Design review of the part built by this model. Coordinates are the model's own, in mm. Coordinates: 2 decimals unless noted, no trailing zeros. Write each loop counter-clockwise with the first axis right and the second up, starting at its lowest first coordinate (ties: lowest second). Pieces come first, ordered by that corner, then holes.
Q1. Add section B-B, the plane x = -28. Give the boundary of the cut face in (y, z), plus the area to 3 significant figures.
Q2. Clearance check with flat-ended pins moving along their axes: pin 1 Ø7 at (x, y) = (-167.8, -27.61) entering from -Z; pin 2 Ø0.9 at (x, z) = (-206, 2) entering from +Y. State where each tip first meets the part, or that it passes through.
Q3. Add section A-A, the plane y = 4. Give the boundary of the cut face in (x, z), plus the area to 3 significant figures.
Q4. To check wall thickness, follow probe 1 along X at (y, z) = (-95.5, 0.9); probe 2 along X at (y, z) = (-38, 0.3); probe 3 along X at (y, z) = (-98, 0.55). State the ranges of each line that lie inside material, in increasing order.
Q5. Add section C-C, the plane z = 2.35. Give the number of separate pieces and of enclosed holes in the cut face, plus the area to 3 significant figures.
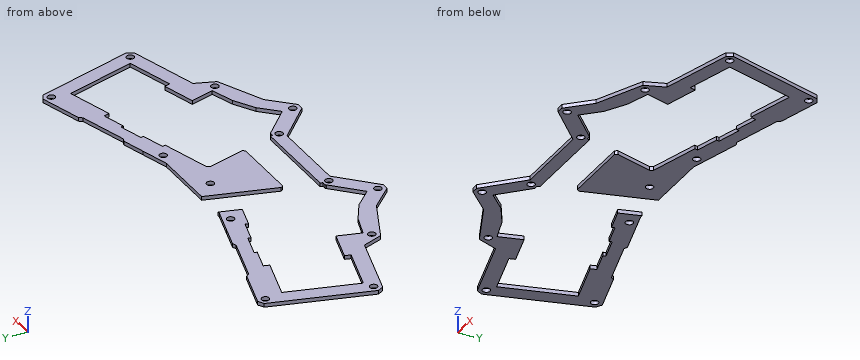
from build123d import *

# Parameters (mm, degrees)
ESQUISSE1_R        = 3
BOSS_EXTRU_1_DEPTH = 3


with BuildPart() as part:
    # Esquisse1 → Boss.-Extru.1 (new body)
    with BuildSketch(Plane.XY):
        Polygon((-106.057456456, -118.225792128), (-128.0696158, -96.878899722), (-131.150893181, -96.85509979), (-131.678504691, -95.01509979), (-203.912015052, -95.01509979), (-204.439626562, -96.85509979), (-207.491865187, -96.85509979), (-208.236606037, -97.572971364), (-229.533063287, -118.225792128), (-242.655085998, -104.673746846), (-258.969310369, -95.012679745), (-277.629290011, -88.825419148), (-272.289144354, -70.202118055), (-298.538981418, -62.6750984), (-299.849714513, -67.246167925), (-337.461409717, -56.461187875), (-321.404434006, -0.463858857), (-284.873898651, -10.938821309), (-283.564528344, -6.372504389), (-265.299260667, -11.609985616), (-264.679553884, -9.448811229), (-245.452786066, -14.960840928), (-246.072799476, -17.123084647), (-227.807531798, -22.360565873), (-228.496674065, -24.763890567), (-209.275142378, -30.275576085), (-204.522611526, -13.701531345), (-206.306232172, -13.701531345), (-228.687205955, -7.283890384), (-246.894010665, -2.064269008), (-249.872259625, -3.248768002), (-288.323340616, 7.774587685), (-290.221637422, 10.357120157), (-324.023652204, 20.047657387), (-328.759186056, 17.422535954), (-351.248940808, -61.008559605), (-348.624077987, -65.743937486), (-292.570685007, -81.816989279), (-286.703799003, -97.823971184), (-249.693611115, -114.655437515), (-232.462472657, -132.451258614), (-227.051679806, -132.536382762), (-198.975350278, -105.350948678), (-136.615169465, -105.350948678), (-108.538839937, -132.536382762), (-103.128047086, -132.451258614), (-85.896908628, -114.655437515), (-48.88672074, -97.823971184), (-43.019834736, -81.816989279), (13.033558244, -65.743937486), (15.658421065, -61.008559605), (-6.831333687, 17.422535954), (-11.566867539, 20.047657387), (-45.368882322, 10.357120157), (-47.267179127, 7.774587685), (-85.718260118, -3.248768002), (-88.696509078, -2.064269008), (-106.903313789, -7.283890384), (-129.284287571, -13.701531345), (-180.595724501, -13.701531345), (-196.24658732, -68.282576398), (-194.797862031, -70.20509979), (-140.792657712, -70.20509979), (-139.343932423, -68.282576398), (-147.87312166, -38.537758661), (-146.501872979, -36.063960558), (-107.093845678, -24.763890567), (-107.782987945, -22.360565873), (-89.517720268, -17.123084647), (-90.137733677, -14.960840928), (-70.910965859, -9.448811229), (-70.291259076, -11.609985616), (-52.025991399, -6.372504389), (-50.716621092, -10.938821309), (-14.186085737, -0.463858857), (1.870889973, -56.461187875), (-35.740805231, -67.246167925), (-37.051538325, -62.6750984), (-63.301375389, -70.202118055), (-57.961229733, -88.825419148), (-76.621209374, -95.012679745), (-92.935433745, -104.673746846), align=None)
        with Locations((-281.934339477, -93.401689518)):
            Circle(ESQUISSE1_R, mode=Mode.SUBTRACT)
        with Locations((-229.666591606, -126.713325795)):
            Circle(ESQUISSE1_R, mode=Mode.SUBTRACT)
        with Locations((-204.059552706, -101.880200807)):
            Circle(ESQUISSE1_R, mode=Mode.SUBTRACT)
        with Locations((-344.882804027, -60.574933915)):
            Circle(ESQUISSE1_R, mode=Mode.SUBTRACT)
        with Locations((-105.923928137, -126.713325795)):
            Circle(ESQUISSE1_R, mode=Mode.SUBTRACT)
        with Locations((-131.530967037, -101.880200807)):
            Circle(ESQUISSE1_R, mode=Mode.SUBTRACT)
        with Locations((-53.656180266, -93.401689518)):
            Circle(ESQUISSE1_R, mode=Mode.SUBTRACT)
        with Locations((9.292284284, -60.574933915)):
            Circle(ESQUISSE1_R, mode=Mode.SUBTRACT)
        with Locations((-323.590068827, 13.68165837)):
            Circle(ESQUISSE1_R, mode=Mode.SUBTRACT)
        with Locations((-216.832585966, -16.924131519)):
            Circle(ESQUISSE1_R, mode=Mode.SUBTRACT)
        with Locations((-118.757933777, -16.924131519)):
            Circle(ESQUISSE1_R, mode=Mode.SUBTRACT)
        with Locations((-12.000450916, 13.68165837)):
            Circle(ESQUISSE1_R, mode=Mode.SUBTRACT)
        with Locations((-167.795259872, -27.605548894)):
            Circle(ESQUISSE1_R, mode=Mode.SUBTRACT)
    extrude(amount=BOSS_EXTRU_1_DEPTH)


solid = part.part
Here are the results:
1. outline: (-77.51, 0) - (-65.03, 0) - (-65.03, 3) - (-77.51, 3) - close; (-4.42, 0) - (15.34, 0) - (15.34, 3) - (-4.42, 3) - close
1. area: 96.7 mm2
2. pin 1: stops at z = 0
2. pin 2: stops at y = -13.66
3. outline: (-332.61, 0) - (-275.16, 0) - (-275.16, 3) - (-332.61, 3) - close; (-60.43, 0) - (-2.98, 0) - (-2.98, 3) - (-60.43, 3) - close
3. area: 345 mm2
4. probe 1: x = -287.56 to -284.08, -279.79 to -258.15, -204.05 to -131.54, -77.44 to -55.8, -51.51 to -48.03
4. probe 2: x = -344.65 to -332.17, -187.56 to -147.58, -3.42 to 9.06
4. probe 3: x = -286.32 to -253.92, -208.68 to -126.91, -81.67 to -49.27
5. separate pieces: 1
5. enclosed holes: 13
5. area: 13,400 mm2
